Could you check a few things on this model? Use its own coordinates, in mm. A direction names the side the tool comes from. Round coordinates to 2 decimals unless told otherwise and drop trailing zeros. Write each loop counter-clockwise with the first axis right and the second up, starting at its lowest first coordinate (ties: lowest second). Pieces come first, ordered by that corner, then holes. Notation, with made-up numbers: (15.25, 32) - (56.25, 32) arc R13 ccw to (56.25, 57) - close; hole circle Ø7 at (-34, -37.5). An arc over 180 degrees is marked (long way). Write each question's results on one line, items separated by ' | '. Start each with the question number.
(1) On a 3-axis mill with a long thin cutter (end or side, diameter ignored), from which of +Z, -Z, +X, -X, +Y, -Y can I reach the whole of each face in a straight line? I mean faces 5 (the flat face through (-1.5, 17.5, -1.2)), 6 (the flat face through (-0.1, 5, 9.7)), 7 (the cylindrical face through (-1.587, 13.525, -2.81)), 8 (the flat face through (0, 11, -5)). Say none if no direction works.
(2) Imagine slicing it at C-C on x = 0. Write out the boundary of the cut face in (y, z).
(3) For P1, Ø4.5, axis at x = 1, z = -12, coming from the +Y side; P2, Ø1, axis at x = 5, y = 11.5, coming from the -Z side, each with a flat end and sliding along its axis, tell me the tip position at first contact or that it passes through.
(4) Thinking about a two-plate mould opening in X: for faces 1 (the cylindrical face through (-0.011, 11.706, 3.322)), 2 (the flat face through (-0.1, 5, -9.8)), 3 (the cylindrical face through (1.587, 13.475, -2.81)), 4 (the flat face through (-6.25, 7, 0)), which applies, +X half, -X half, draft (parallel to the pull), parting line (faces both ways), or undercut?
(5) Imagine slicing it at A-A on z = 0. Write out the boundary of the cut face in (x, y).
(6) Imagine slicing it at D-D on y = 4.25. Write out the boundary of the cut face in (x, z), then the cut area to 3 significant figures.
(7) Please list where these lines run through material, in increasing order: line 1 (Z direction, x = 0, y = 6.75); line 2 (X direction, y = 12, z = 0); line 3 (X direction, y = 4, z = 11.5). Write a range as [from, to].
(8) Imagine slicing it at B-B on y = 10.25. Write out the boundary of the cut face in (x, z), then the cut area to 3 significant figures.
```python
from build123d import *

# Parameters (mm, degrees)
SKETCH1_W                          = 12.5
SKETCH1_H                          = 28.9
EXTRUDE1_DEPTH                     = 5
F_3_0_3_DIAMETER_HOLE1_D           = 3
SKETCH5_W                          = 12.5
SKETCH5_H                          = 10
EXTRUDE3_DEPTH                     = 12.5
F_1_8_0_125_DIAMETER_HOLE1_D       = 3.175
F_8_32_TAPPED_HOLE1_D              = 3.4544
F_8_32_TAPPED_HOLE1_ON_FACE_2_D    = 3.4544
F_1_16_0_0625_DIAMETER_HOLE2_D     = 1.5875
F_1_16_0_0625_DIAMETER_HOLE2_DEPTH = 19.45
F_1_16_0_0625_DIAMETER_HOLE2_TIP   = 0.476933116


with BuildPart() as part:
    # Sketch1 → Extrude1 (new body)
    with BuildSketch(Plane(origin=(0, 0, 0), x_dir=(1, 0, 0), z_dir=(0, 1, 0))):
        Rectangle(SKETCH1_W, SKETCH1_H)
    extrude(amount=EXTRUDE1_DEPTH)

    # Ø3.0 (3) Diameter Hole1 (through all)
    with Locations(Plane(origin=(0, 5, -11.45), x_dir=(0, 0, 1), z_dir=(0, 1, 0))):
        with Locations((0, 0), (22.9, 0)):
            Hole(F_3_0_3_DIAMETER_HOLE1_D / 2)

    # Sketch5 → Extrude3 (add)
    with BuildSketch(Plane(origin=(0, 5, 0), x_dir=(1, 0, 0), z_dir=(0, 1, 0))):
        Rectangle(SKETCH5_W, SKETCH5_H)
    extrude(amount=EXTRUDE3_DEPTH)

    # 1/8 (0.125) Diameter Hole1 (through all)
    with Locations(Plane(origin=(0, 13.5, -5), x_dir=(-1, 0, 0), z_dir=(0, 0, -1))):
        with Locations((0, 0)):
            Hole(F_1_8_0_125_DIAMETER_HOLE1_D / 2)

    # #8-32 Tapped Hole1 (through all)
    with Locations(Plane.ZX.offset(17.5)):
        with Locations((0, 0)):
            Hole(F_8_32_TAPPED_HOLE1_D / 2)

    # #8-32 Tapped Hole1 on face 2 (through all)
    with Locations(Plane(origin=(0, 0, 0), x_dir=(0, 0, -1), z_dir=(0, -1, 0))):
        with Locations((0, 0)):
            Hole(F_8_32_TAPPED_HOLE1_ON_FACE_2_D / 2)

    # 1/16 (0.0625) Diameter Hole2
    with Locations(Plane(origin=(0, 14.5, -5), x_dir=(-1, 0, 0), z_dir=(0, 0, -1))):
        with Locations((0, 0), (0, -2)):
            Hole(F_1_16_0_0625_DIAMETER_HOLE2_D / 2, depth=F_1_16_0_0625_DIAMETER_HOLE2_DEPTH)
            with Locations((0, 0, -(F_1_16_0_0625_DIAMETER_HOLE2_DEPTH + F_1_16_0_0625_DIAMETER_HOLE2_TIP / 2))):  # 118° drill point
                Cone(0, F_1_16_0_0625_DIAMETER_HOLE2_D / 2, F_1_16_0_0625_DIAMETER_HOLE2_TIP, mode=Mode.SUBTRACT)


solid = part.part
```
Response:
1) face 5: +Z, -Z, +X, -X, +Y | face 6: +Z, +X, -X, +Y | face 7: +Z, -Z | face 8: -Z, +X, -X, +Y
2) outline: (0, -14.45) - (5, -14.45) - (5, -12.95) - (0, -12.95) - close; (0, -9.95) - (5, -9.95) - (5, -5) - (11.71, -5) - (11.71, -1.73) - (0, -1.73) - close; (0, 1.73) - (11.71, 1.73) - (11.71, 5) - (5, 5) - (5, 9.95) - (0, 9.95) - close; (0, 12.95) - (5, 12.95) - (5, 14.45) - (0, 14.45) - close; (15.29, -5) - (17.5, -5) - (17.5, -1.73) - (15.29, -1.73) - close; (15.29, 1.73) - (17.5, 1.73) - (17.5, 5) - (15.29, 5) - close
3) P1: y = 5 | P2: z = -5
4) face 1: undercut | face 2: draft | face 3: undercut | face 4: -X half
5) outline: (-6.25, 0) - (-1.73, 0) - (-1.73, 17.5) - (-6.25, 17.5) - close; (1.73, 0) - (6.25, 0) - (6.25, 17.5) - (1.73, 17.5) - close
6) outline: (-6.25, -14.45) - (6.25, -14.45) - (6.25, 14.45) - (-6.25, 14.45) - close; hole circle Ø3.45 at (0, 0); hole circle Ø3 at (0, -11.45); hole circle Ø3 at (0, 11.45) | area: 338 mm²
7) line 1: [-5, -1.73], [1.73, 5] | line 2: [-6.25, -1.73], [1.73, 6.25] | line 3: [-6.25, -1.5], [1.5, 6.25]
8) outline: (-6.25, -5) - (6.25, -5) - (6.25, 5) - (-6.25, 5) - close; hole circle Ø3.45 at (0, 0) | area: 116 mm²
